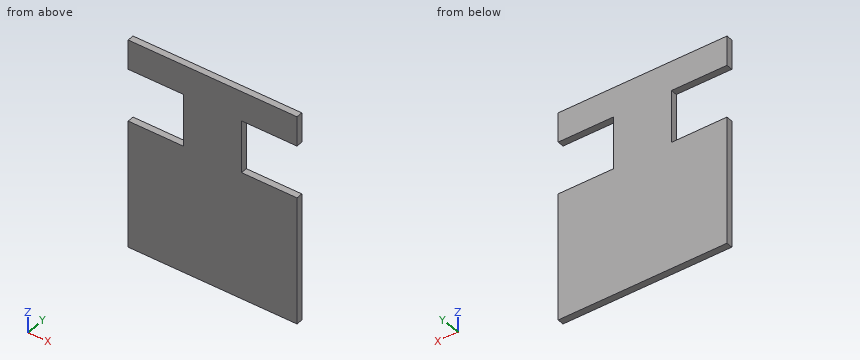
Autodesk Inventor part; units mm, degrees
ref_plane "XZ Plane" through (0, 0, 0) normal (0, 1, 0) x (-1, 0, 0)
ref_plane "XY Plane" through (0, 0, 0) normal (0, 0, 1) x (1, 0, 0)
sketch "Sketch1" plane through (0, 0, 0) normal (0, 1, 0) x (-1, 0, 0)
  line L0 (-231.775, 292.1) -> (-231.775, -292.1)
  line L1 (-231.775, -292.1) -> (231.775, -292.1)
  line L2 (231.775, -292.1) -> (231.775, 292.1)
  line L3 (231.775, 292.1) -> (-231.775, 292.1)
  line L4 (-231.775, 292.1) -> (231.775, -292.1) construction
  line L5 (-231.775, -292.1) -> (231.775, 292.1) construction
  point P0 (0, 0)
  dimension "baseLength" = 584.2
  dimension "baseWidth" = 463.55
extrude "Extrusion1" add sketch "Sketch1" along normal blind 17.78
sketch "Sketch2" plane through (0, 0, 0) normal (0, -1, 0) x (1, 0, 0)
  line L0 (231.775, 292.1) -> (231.775, -292.1)
  line L1 (231.775, 209.55) -> (79.375, 209.55)
  line L2 (79.375, 209.55) -> (79.375, 63.5)
  line L3 (79.375, 63.5) -> (231.775, 63.5)
  line L4 (231.775, 63.5) -> (231.775, 209.55)
  line L5 (-231.775, 292.1) -> (231.775, 292.1)
  point P0 (0, 0)
  dimension "backToEndOfGearBox" = 82.55
  dimension "backToFrontOfGearBox" = 228.6
  dimension "wdithForGearBox" = 152.4
extrude "Extrusion2" cut sketch "Sketch2" against normal through all
mirror "Mirror1" about plane through (0, 0, 0) normal (1, 0, 0) of "Extrusion2"
equation "\"spaceingAlongSides\" = 3.175"
equation "\"distanceFromBackForEndBolt\" = 38.1"
equation "\"spacingForBolt\" = 25.4"
equation "\"widthOfSpacingForBolt\" = 12.7"
equation "\"lengthOfSpacingForBolt\" = 25.4"
properties part number "RhinoBottomFloorPlate02" material "Wood (Birch)"
CAD build for the part. Positions are in the model's coordinates, mm. Give positions to 0.01 mm unless a question says otherwise; leave off trailing zeros. Order: outer loops, then holes, each group sorted by start corner. A loop starts at its lowest first (then second) coordinate and runs counter-clockwise, first axis right, second up.
(1) Drill centre lines: L1, parallel to Z at x = -92, y = 11; L2, parallel to X at y = 10.5, z = 171.5 (3 decimals). Where is each one in solid material? Low to high.
(2) Flat gauge pins, fed straight in: pin 1 (5 mm diameter, centred on y = 7, z = 74.5, fed in from +X) (3 decimals); pin 2 (6 mm diameter, centred on y = 8, z = 122, fed in from -X) (3 decimals); pin 3 (10 mm diameter, centred on x = -21.5, z = 71, fed in from -Y). Where does each tip first touch, or does it go through?
(3) Saw through at A-A, the plane x = -158. Give the cut face in (y, z), then the cut area to 3 significant figures.
(4) Saw through at C-C, the plane z = 112.5. Give the cut face in (x, y) (3 decimals), then the cut area to 3 significant figures.
(5) Saw through at B-B, the plane y = 13.5. Give the cut face in (x, z) (3 decimals), then the cut area to 3 significant figures.
Results found:
1. L1: z = -292.1 to 63.5, 209.55 to 292.1
1. L2: x = -79.375 to 79.375
2. pin 1: stops at x = 79.375
2. pin 2: stops at x = -79.375
2. pin 3: stops at y = 0
3. outline: (0, -292.1) - (17.78, -292.1) - (17.78, 63.5) - (0, 63.5) - close; (0, 209.55) - (17.78, 209.55) - (17.78, 292.1) - (0, 292.1) - close
3. area: 7,790 mm2
4. outline: (-79.375, 0) - (79.375, 0) - (79.375, 17.78) - (-79.375, 17.78) - close
4. area: 2,820 mm2
5. outline: (-231.775, -292.1) - (231.775, -292.1) - (231.775, 63.5) - (79.375, 63.5) - (79.375, 209.55) - (231.775, 209.55) - (231.775, 292.1) - (-231.775, 292.1) - (-231.775, 209.55) - (-79.375, 209.55) - (-79.375, 63.5) - (-231.775, 63.5) - close
5. area: 226,000 mm2
